```python
from build123d import *

# Parameters (mm, degrees)
F0_W     = 82.2
F0_H     = 62.4
F0_R     = 1.5
F0_R_2   = 9.4
F0_W_2   = 3
F0_H_2   = 1.1
F0_R_3   = 3
F0_R_4   = 2
F1_DEPTH = 4
F2_R     = 3


with BuildPart() as f1:
    # F0 (on Front) → F1 (new body)
    with BuildSketch(Plane.XZ):
        with Locations((29.7, 19.8)):
            Rectangle(F0_W, F0_H)
        with Locations((-8.630646, -8.630646)):
            Circle(F0_R, mode=Mode.SUBTRACT)
        Circle(F0_R_2, mode=Mode.SUBTRACT)
        with Locations((9.9, -9.6)):
            Rectangle(F0_W_2, F0_H_2, mode=Mode.SUBTRACT)
        with Locations((9.9, -7)):
            Rectangle(F0_W_2, F0_H_2, mode=Mode.SUBTRACT)
        with Locations((19.8, 0)):
            Circle(F0_R_2, mode=Mode.SUBTRACT)
        with Locations((-8.630646, 9.9)):
            Circle(F0_R, mode=Mode.SUBTRACT)
        with Locations((9.9, 9.9)):
            Circle(F0_R_3, mode=Mode.SUBTRACT)
        with Locations((29.7, -8.425556)):
            Circle(F0_R_4, mode=Mode.SUBTRACT)
        with Locations((49.5, -9.6)):
            Rectangle(F0_W_2, F0_H_2, mode=Mode.SUBTRACT)
        with Locations((49.5, -7)):
            Rectangle(F0_W_2, F0_H_2, mode=Mode.SUBTRACT)
        with Locations((39.6, 0)):
            Circle(F0_R_2, mode=Mode.SUBTRACT)
        with Locations((68.030646, -8.630646)):
            Circle(F0_R, mode=Mode.SUBTRACT)
        with Locations((59.4, 0)):
            Circle(F0_R_2, mode=Mode.SUBTRACT)
        with Locations((29.7, 9.9)):
            Circle(F0_R_3, mode=Mode.SUBTRACT)
        with Locations((49.5, 9.9)):
            Circle(F0_R_3, mode=Mode.SUBTRACT)
        with Locations((68.030646, 9.9)):
            Circle(F0_R, mode=Mode.SUBTRACT)
        with Locations((0, 19.8)):
            Circle(F0_R_2, mode=Mode.SUBTRACT)
        with Locations((-8.630646, 29.7)):
            Circle(F0_R, mode=Mode.SUBTRACT)
        with Locations((19.8, 19.8)):
            Circle(F0_R_2, mode=Mode.SUBTRACT)
        with Locations((9.9, 29.7)):
            Circle(F0_R_3, mode=Mode.SUBTRACT)
        with Locations((0, 39.6)):
            Circle(F0_R_2, mode=Mode.SUBTRACT)
        with Locations((-8.630646, 48.230646)):
            Circle(F0_R, mode=Mode.SUBTRACT)
        with Locations((19.8, 39.6)):
            Circle(F0_R_2, mode=Mode.SUBTRACT)
        with Locations((9.9, 46.6)):
            Rectangle(F0_W_2, F0_H_2, mode=Mode.SUBTRACT)
        with Locations((9.9, 49.2)):
            Rectangle(F0_W_2, F0_H_2, mode=Mode.SUBTRACT)
        with Locations((39.6, 19.8)):
            Circle(F0_R_2, mode=Mode.SUBTRACT)
        with Locations((29.7, 29.7)):
            Circle(F0_R_3, mode=Mode.SUBTRACT)
        with Locations((49.5, 29.7)):
            Circle(F0_R_3, mode=Mode.SUBTRACT)
        with Locations((59.4, 19.8)):
            Circle(F0_R_2, mode=Mode.SUBTRACT)
        with Locations((68.030646, 29.7)):
            Circle(F0_R, mode=Mode.SUBTRACT)
        with Locations((39.6, 39.6)):
            Circle(F0_R_2, mode=Mode.SUBTRACT)
        with Locations((29.7, 48.025556)):
            Circle(F0_R_4, mode=Mode.SUBTRACT)
        with Locations((49.5, 46.6)):
            Rectangle(F0_W_2, F0_H_2, mode=Mode.SUBTRACT)
        with Locations((49.5, 49.2)):
            Rectangle(F0_W_2, F0_H_2, mode=Mode.SUBTRACT)
        with Locations((59.4, 39.6)):
            Circle(F0_R_2, mode=Mode.SUBTRACT)
        with Locations((68.030646, 48.230646)):
            Circle(F0_R, mode=Mode.SUBTRACT)
    extrude(amount=F1_DEPTH)

    # F2
    f2_edges = [f1.edges().sort_by_distance(p)[0] for p in [
        (70.8, -2, 51),
        (-11.4, -2, 51),
        (-11.4, -2, -11.4),
        (70.8, -2, -11.4),
    ]]
    fillet(f2_edges, radius=F2_R)


solid = f1.part
```
Source: CAD feature listing. Evaluate the final solid. Frame: model axes, mm. A direction names the side the tool comes from. Round coordinates to 2 decimals unless told otherwise and drop trailing zeros. Loops run counter-clockwise (first coordinate to the right, second up) from the corner with the lowest first, then second, coordinate; pieces in that order, holes last. Notation, with made-up numbers: M 64.5,-4.75 L 73.5,-4.75 A15 ccw 73.5,17.25 Z; hole C 29.5,48 d2. An arc over 180 degrees is marked long. Use a Markdown table: item, result. Add a question column.
1. Pull-direction query (X, two-part tool) for faces 1 (the cylindrical face through (69.9, -2.03, 50.14)), 2 (the flat face through (30, -4, 20)), 3 (the cylindrical face through (24.85, -1.97, 27.73)); classes: +X half, -X half, draft (parallel to the pull), parting line (faces both ways), or undercut.
2. Ray query, line 1 along Z through (x, y) = (19.8, -1.65); line 2 along X through (y, z) = (-1, 0.5); line 3 along X through (y, z) = (-2.5, 3.5). Return the intervals inside material, ascending. Write a range as [from, to].
3. Cut plane A-A, the plane x = 19.8. Output: boundary loops of the cut face in (y, z).
4. Set-up query: faces 4 (the flat face through (49, -2, 48.65)), 5 (the flat face through (29, -2, 51)). Return all of +Z, -Z, +X, -X, +Y, -Y with unobstructed straight access to the full face (end or side cutting, diameter ignored); none if empty.
5. Contact query for a flat-ended pin moving along its axis: pin 1 (1.2 mm diameter, centred on y = -1, z = 49.5, fed in from +X). Output: stop coordinate, or through.
6. Cut plane C-C, the plane z = -2. Output: boundary loops of the cut face in (x, y), and give its area (3 significant figures).
7. Cut plane D-D, the plane y = -1.3. State how many separate pieces and enclosed holes the cut face has, and give its area (3 significant figures).
8. Cut plane B-B, the plane z = 39.6. Output: boundary loops of the cut face in (x, y), and give its area (3 significant figures).
Solution:
| question | item | result |
|---|---|---|
| 1 | face 1 | +X half |
| 1 | face 2 | draft |
| 1 | face 3 | undercut |
| 2 | line 1 | z = [-11.4, -9.4], [9.4, 10.4], [29.2, 30.2], [49, 51] |
| 2 | line 2 | x = [-11.4, -9.39], [9.39, 10.41], [29.19, 30.21], [48.99, 50.01], [68.79, 70.8] |
| 2 | line 3 | x = [-11.4, -8.72], [8.72, 11.08], [28.52, 30.88], [48.32, 50.68], [68.12, 70.8] |
| 3 | outline | M -4,-11.4 L 0,-11.4 L 0,-9.4 L -4,-9.4 Z; M -4,9.4 L 0,9.4 L 0,10.4 L -4,10.4 Z; M -4,29.2 L 0,29.2 L 0,30.2 L -4,30.2 Z; M -4,49 L 0,49 L 0,51 L -4,51 Z |
| 4 | face 4 | +Y, -Y |
| 4 | face 5 | +Z, +X, -X, +Y, -Y |
| 5 | pin 1 | stops at x = 70.66 |
| 6 | outline | M -11.4,-4 L -9.18,-4 L -9.18,0 L -11.4,0 Z; M 9.18,-4 L 10.62,-4 L 10.62,0 L 9.18,0 Z; M 28.98,-4 L 30.42,-4 L 30.42,0 L 28.98,0 Z; M 48.78,-4 L 50.22,-4 L 50.22,0 L 48.78,0 Z; M 68.58,-4 L 70.8,-4 L 70.8,0 L 68.58,0 Z |
| 6 | area | 34.9 mm2 |
| 7 | separate pieces | 1 |
| 7 | enclosed holes | 36 |
| 7 | area | 1,510 mm2 |
| 8 | outline | M -11.4,-4 L -9.4,-4 L -9.4,0 L -11.4,0 Z; M 9.4,-4 L 10.4,-4 L 10.4,0 L 9.4,0 Z; M 29.2,-4 L 30.2,-4 L 30.2,0 L 29.2,0 Z; M 49,-4 L 50,-4 L 50,0 L 49,0 Z; M 68.8,-4 L 70.8,-4 L 70.8,0 L 68.8,0 Z |
| 8 | area | 28.0 mm2 |
